from build123d import *

# Parameters (mm, degrees)
SKETCH_2_W              = 70
SKETCH_2_H              = 50
SKETCH_2_R              = 1.75
EXTRUDE_1_DEPTH         = 1
SKETCH_3_W              = 51
SKETCH_3_H              = 2.5
EXTRUDE_2_DEPTH         = 8.4
SKETCH_4_W              = 10.16
SKETCH_4_H              = 2.54
EXTRUDE_3_DEPTH         = 2
SKETCH_5_R              = 0.5
EXTRUDE_4_DEPTH         = 6
SKETCH_6_W              = 7
SKETCH_6_H              = 7
EXTRUDE_5_DEPTH         = 10
CHAMFER_1_SIZE          = 5
CHAMFER_1_SIZE2         = 1.339745962
CHAMFER_1_PART_2_SIZE   = 5
CHAMFER_1_PART_2_SIZE2  = 1.339745962
CHAMFER_1_PART_3_SIZE   = 5
CHAMFER_1_PART_3_SIZE2  = 1.339745962
CHAMFER_1_PART_4_SIZE   = 5
CHAMFER_1_PART_4_SIZE2  = 1.339745962
CHAMFER_1_PART_5_SIZE   = 5
CHAMFER_1_PART_5_SIZE2  = 1.339745962
CHAMFER_1_PART_6_SIZE   = 5
CHAMFER_1_PART_6_SIZE2  = 1.339745962
CHAMFER_1_PART_7_SIZE   = 5
CHAMFER_1_PART_7_SIZE2  = 1.339745962
CHAMFER_1_PART_8_SIZE   = 5
CHAMFER_1_PART_8_SIZE2  = 1.339745962
CHAMFER_1_PART_9_SIZE   = 5
CHAMFER_1_PART_9_SIZE2  = 1.339745962
CHAMFER_1_PART_10_SIZE  = 5
CHAMFER_1_PART_10_SIZE2 = 1.339745962
CUT_EXTRUDE_START       = 0.046624
SKETCH_7_R              = 1
CUT_EXTRUDE_1_DEPTH     = 2


with BuildPart() as part:
    # Эскиз2 → Бобышка-Вытянуть1 (new body)
    with BuildSketch(Plane(origin=(0, 0, 0), x_dir=(1, 0, 0), z_dir=(0, 1, 0))):
        with Locations((35, 25)):
            Rectangle(SKETCH_2_W, SKETCH_2_H)
        with Locations((5, 45)):
            Circle(SKETCH_2_R, mode=Mode.SUBTRACT)
        with Locations((65, 45)):
            Circle(SKETCH_2_R, mode=Mode.SUBTRACT)
        with Locations((65, 5)):
            Circle(SKETCH_2_R, mode=Mode.SUBTRACT)
        with Locations((5, 5)):
            Circle(SKETCH_2_R, mode=Mode.SUBTRACT)
    extrude(amount=EXTRUDE_1_DEPTH)

    # Эскиз3 → Бобышка-Вытянуть2 (add)
    with BuildSketch(Plane(origin=(0, 1, 0), x_dir=(1, 0, 0), z_dir=(0, 1, 0))):
        with Locations((34.5, 11.25)):
            Rectangle(SKETCH_3_W, SKETCH_3_H)
        with Locations((34.5, 26.75)):
            Rectangle(SKETCH_3_W, SKETCH_3_H)
    extrude(amount=EXTRUDE_2_DEPTH)

    # Эскиз4 → Бобышка-Вытянуть3 (add)
    with BuildSketch(Plane(origin=(0, 1, 0), x_dir=(1, 0, 0), z_dir=(0, 1, 0))):
        with Locations((54.92, 4.27)):
            Rectangle(SKETCH_4_W, SKETCH_4_H)
        with Locations((42.92, 4.27)):
            Rectangle(SKETCH_4_W, SKETCH_4_H)
        with Locations((15.08, 4.27)):
            Rectangle(SKETCH_4_W, SKETCH_4_H)
        with Locations((27.08, 4.27)):
            Rectangle(SKETCH_4_W, SKETCH_4_H)
        with Locations((58.562253528, 38.283187026)):
            Rectangle(SKETCH_4_W, SKETCH_4_H)
        with Locations((58.594566993, 33.283187026)):
            Rectangle(SKETCH_4_W, SKETCH_4_H)
    extrude(amount=EXTRUDE_3_DEPTH)

    # Эскиз5 → Бобышка-Вытянуть4 (add)
    with BuildSketch(Plane(origin=(0, 3, 0), x_dir=(1, 0, 0), z_dir=(0, 1, 0))):
        with Locations((58.73, 4.27)):
            Circle(SKETCH_5_R)
        with Locations((56.19, 4.27)):
            Circle(SKETCH_5_R)
        with Locations((53.65, 4.27)):
            Circle(SKETCH_5_R)
        with Locations((51.11, 4.27)):
            Circle(SKETCH_5_R)
        with Locations((46.73, 4.27)):
            Circle(SKETCH_5_R)
        with Locations((44.19, 4.27)):
            Circle(SKETCH_5_R)
        with Locations((41.65, 4.27)):
            Circle(SKETCH_5_R)
        with Locations((39.11, 4.27)):
            Circle(SKETCH_5_R)
        with Locations((25.81, 4.27)):
            Circle(SKETCH_5_R)
        with Locations((11.27, 4.27)):
            Circle(SKETCH_5_R)
        with Locations((13.81, 4.27)):
            Circle(SKETCH_5_R)
        with Locations((16.35, 4.27)):
            Circle(SKETCH_5_R)
        with Locations((18.89, 4.27)):
            Circle(SKETCH_5_R)
        with Locations((23.27, 4.27)):
            Circle(SKETCH_5_R)
        with Locations((28.35, 4.27)):
            Circle(SKETCH_5_R)
        with Locations((30.89, 4.27)):
            Circle(SKETCH_5_R)
        with Locations((54.67096141, 33.208395661)):
            Circle(SKETCH_5_R)
        with Locations((54.67096141, 38.208395661)):
            Circle(SKETCH_5_R)
        with Locations((57.21096141, 33.208395661)):
            Circle(SKETCH_5_R)
        with Locations((59.75096141, 33.208395661)):
            Circle(SKETCH_5_R)
        with Locations((62.29096141, 33.208395661)):
            Circle(SKETCH_5_R)
        with Locations((57.21096141, 38.208395661)):
            Circle(SKETCH_5_R)
        with Locations((59.75096141, 38.208395661)):
            Circle(SKETCH_5_R)
        with Locations((62.29096141, 38.208395661)):
            Circle(SKETCH_5_R)
    extrude(amount=EXTRUDE_4_DEPTH)

    # Эскиз6 → Бобышка-Вытянуть5 (add)
    with BuildSketch(Plane(origin=(0, 1, 0), x_dir=(1, 0, 0), z_dir=(0, 1, 0))):
        with Locations((23.247184381, 44.500218353)):
            Rectangle(SKETCH_6_W, SKETCH_6_H)
        with Locations((11.946306787, 44.453594358)):
            Rectangle(SKETCH_6_W, SKETCH_6_H)
        with Locations((33.247184381, 44.500218353)):
            Rectangle(SKETCH_6_W, SKETCH_6_H)
        with Locations((43.247184381, 44.500218353)):
            Rectangle(SKETCH_6_W, SKETCH_6_H)
        with Locations((53.247184381, 44.500218353)):
            Rectangle(SKETCH_6_W, SKETCH_6_H)
    extrude(amount=EXTRUDE_5_DEPTH)

    # Фаска1
    chamfer_1_edges = [part.edges().sort_by_distance(p)[0] for p in [
        (23.247184381, 11, -41.000218353),
    ]]
    chamfer_1_side = [part.faces().sort_by_distance(p)[0] for p in [
        (23.247184381, 6, -41.000218353),
    ]]
    chamfer(chamfer_1_edges, length=CHAMFER_1_SIZE, length2=CHAMFER_1_SIZE2, reference=chamfer_1_side[0])

    # Фаска1 part 2
    chamfer_1_part_2_edges = [part.edges().sort_by_distance(p)[0] for p in [
        (23.247184381, 11, -48.000218353),
    ]]
    chamfer_1_part_2_side = [part.faces().sort_by_distance(p)[0] for p in [
        (23.247184381, 6, -48.000218353),
    ]]
    chamfer(chamfer_1_part_2_edges, length=CHAMFER_1_PART_2_SIZE, length2=CHAMFER_1_PART_2_SIZE2, reference=chamfer_1_part_2_side[0])

    # Фаска1 part 3
    chamfer_1_part_3_edges = [part.edges().sort_by_distance(p)[0] for p in [
        (11.946306787, 11, -40.953594358),
    ]]
    chamfer_1_part_3_side = [part.faces().sort_by_distance(p)[0] for p in [
        (11.946306787, 6, -40.953594358),
    ]]
    chamfer(chamfer_1_part_3_edges, length=CHAMFER_1_PART_3_SIZE, length2=CHAMFER_1_PART_3_SIZE2, reference=chamfer_1_part_3_side[0])

    # Фаска1 part 4
    chamfer_1_part_4_edges = [part.edges().sort_by_distance(p)[0] for p in [
        (11.946306787, 11, -47.953594358),
    ]]
    chamfer_1_part_4_side = [part.faces().sort_by_distance(p)[0] for p in [
        (11.946306787, 6, -47.953594358),
    ]]
    chamfer(chamfer_1_part_4_edges, length=CHAMFER_1_PART_4_SIZE, length2=CHAMFER_1_PART_4_SIZE2, reference=chamfer_1_part_4_side[0])

    # Фаска1 part 5
    chamfer_1_part_5_edges = [part.edges().sort_by_distance(p)[0] for p in [
        (33.247184381, 11, -41.000218353),
    ]]
    chamfer_1_part_5_side = [part.faces().sort_by_distance(p)[0] for p in [
        (33.247184381, 6, -41.000218353),
    ]]
    chamfer(chamfer_1_part_5_edges, length=CHAMFER_1_PART_5_SIZE, length2=CHAMFER_1_PART_5_SIZE2, reference=chamfer_1_part_5_side[0])

    # Фаска1 part 6
    chamfer_1_part_6_edges = [part.edges().sort_by_distance(p)[0] for p in [
        (33.247184381, 11, -48.000218353),
    ]]
    chamfer_1_part_6_side = [part.faces().sort_by_distance(p)[0] for p in [
        (33.247184381, 6, -48.000218353),
    ]]
    chamfer(chamfer_1_part_6_edges, length=CHAMFER_1_PART_6_SIZE, length2=CHAMFER_1_PART_6_SIZE2, reference=chamfer_1_part_6_side[0])

    # Фаска1 part 7
    chamfer_1_part_7_edges = [part.edges().sort_by_distance(p)[0] for p in [
        (43.247184381, 11, -41.000218353),
    ]]
    chamfer_1_part_7_side = [part.faces().sort_by_distance(p)[0] for p in [
        (43.247184381, 6, -41.000218353),
    ]]
    chamfer(chamfer_1_part_7_edges, length=CHAMFER_1_PART_7_SIZE, length2=CHAMFER_1_PART_7_SIZE2, reference=chamfer_1_part_7_side[0])

    # Фаска1 part 8
    chamfer_1_part_8_edges = [part.edges().sort_by_distance(p)[0] for p in [
        (43.247184381, 11, -48.000218353),
    ]]
    chamfer_1_part_8_side = [part.faces().sort_by_distance(p)[0] for p in [
        (43.247184381, 6, -48.000218353),
    ]]
    chamfer(chamfer_1_part_8_edges, length=CHAMFER_1_PART_8_SIZE, length2=CHAMFER_1_PART_8_SIZE2, reference=chamfer_1_part_8_side[0])

    # Фаска1 part 9
    chamfer_1_part_9_edges = [part.edges().sort_by_distance(p)[0] for p in [
        (53.247184381, 11, -41.000218353),
    ]]
    chamfer_1_part_9_side = [part.faces().sort_by_distance(p)[0] for p in [
        (53.247184381, 6, -41.000218353),
    ]]
    chamfer(chamfer_1_part_9_edges, length=CHAMFER_1_PART_9_SIZE, length2=CHAMFER_1_PART_9_SIZE2, reference=chamfer_1_part_9_side[0])

    # Фаска1 part 10
    chamfer_1_part_10_edges = [part.edges().sort_by_distance(p)[0] for p in [
        (53.247184381, 11, -48.000218353),
    ]]
    chamfer_1_part_10_side = [part.faces().sort_by_distance(p)[0] for p in [
        (53.247184381, 6, -48.000218353),
    ]]
    chamfer(chamfer_1_part_10_edges, length=CHAMFER_1_PART_10_SIZE, length2=CHAMFER_1_PART_10_SIZE2, reference=chamfer_1_part_10_side[0])

    # Эскиз7 → Вырез-Вытянуть1 (cut)
    with BuildSketch(Plane(origin=(0, 0, -47.953594358), x_dir=(-1, 0, 0), z_dir=(0, 0, -1)).offset(CUT_EXTRUDE_START)):
        with Locations((-10.259866322, 3.21835238)):
            Circle(SKETCH_7_R)
        with Locations((-13.281229876, 3.21835238)):
            Circle(SKETCH_7_R)
        with Locations((-21.706301123, 3.223335503)):
            Circle(SKETCH_7_R)
        with Locations((-24.727664678, 3.223335503)):
            Circle(SKETCH_7_R)
        with Locations((-34.727664678, 3.223335503)):
            Circle(SKETCH_7_R)
        with Locations((-31.706301123, 3.223335503)):
            Circle(SKETCH_7_R)
        with Locations((-44.727664678, 3.223335503)):
            Circle(SKETCH_7_R)
        with Locations((-41.706301123, 3.223335503)):
            Circle(SKETCH_7_R)
        with Locations((-54.727664678, 3.223335503)):
            Circle(SKETCH_7_R)
        with Locations((-51.706301123, 3.223335503)):
            Circle(SKETCH_7_R)
    extrude(amount=-CUT_EXTRUDE_1_DEPTH, mode=Mode.SUBTRACT)


solid = part.part
The listing builds one solid part. Answer for the finished solid, in the listing's coordinates (mm). A direction names the side the tool comes from. Coordinates: 2 decimals unless noted, no trailing zeros. Order: outer loops, then holes, each group sorted by start corner. A loop starts at its lowest first (then second) coordinate and runs counter-clockwise, first axis right, second up.
Q1. Which of the six approach directions +Z, -Z, +X, -X, +Y, -Y give full straight-line access (tool end or side, diameter ignored) to faces 4 (the face through (56.747, 6, -44)), 5 (the face through (42, 3, -46)), 6 (the face through (60, 5, -11))?
Q2. Given P1, Ø1.6, axis at x = 41.5, y = 2.5, coming from the -Z side; P2, Ø5, axis at y = 7.5, z = -27, coming from the -X side; P3, Ø2, axis at x = 57.5, z = -33, coming from the +Y side, each flat-ended and moving along its own axis, determine where each tip first touches the part or whether it passes through.
Q3. A cutting plane is placed at B-B, the plane y = 10.25. Write down the section's boundary in (x, z), and give its area (3 significant figures).
Q4. For a pull along Y with two mould halves and no side action, classify faces 1 (the face through (42.44, 3.9, -47.01)), 2 (the face through (53.2, 8.54, -47.32)), 3 (the face through (34, 5, -10)) as pulls with the +Y half, pulls with the -Y half, needs draft (parallel to the pull), parting line crosses it, or undercut.
Q5. A cutting plane is placed at A-A, the plane x = 5. Write down the section's boundary in (y, z), and give its area (3 significant figures).
Q6. A cutting plane is placed at C-C, the plane z = -8.5. Write down the section's boundary in (x, y).
Q7. Consider line 1 (X direction, y = 4.5, z = -44); line 2 (Z direction, x = 50, y = 5); line 3 (X direction, y = 0.35, z = -45). Determine where each line is inside the solid, lowest interval first.
Answers follow:
1. face 4: -Z, +X, +Y
1. face 5: -Z
1. face 6: +Z, +X, +Y
2. P1: stops at z = -48
2. P2: stops at x = 9
2. P3: stops at y = 9
3. outline: (8.45, -46.81) - (15.45, -46.81) - (15.45, -42.09) - (8.45, -42.09) - close; (19.75, -46.86) - (26.75, -46.86) - (26.75, -42.14) - (19.75, -42.14) - close; (29.75, -46.86) - (36.75, -46.86) - (36.75, -42.14) - (29.75, -42.14) - close; (39.75, -46.86) - (46.75, -46.86) - (46.75, -42.14) - (39.75, -42.14) - close; (49.75, -46.86) - (56.75, -46.86) - (56.75, -42.14) - (49.75, -42.14) - close
3. area: 165 mm2
4. face 1: undercut
4. face 2: pulls with the +Y half
4. face 3: needs draft
5. outline: (0, -50) - (1, -50) - (1, -46.75) - (0, -46.75) - close; (0, -43.25) - (1, -43.25) - (1, -6.75) - (0, -6.75) - close; (0, -3.25) - (1, -3.25) - (1, 0) - (0, 0) - close
5. area: 43.0 mm2
6. outline: (0, 0) - (70, 0) - (70, 1) - (0, 1) - close
7. line 1: x = 8.45 to 15.45, 19.75 to 26.75, 29.75 to 36.75, 39.75 to 46.75, 49.75 to 56.75
7. line 2: z = -48 to -41, -28 to -25.5, -12.5 to -10
7. line 3: x = 0 to 3.25, 6.75 to 63.25, 66.75 to 70
